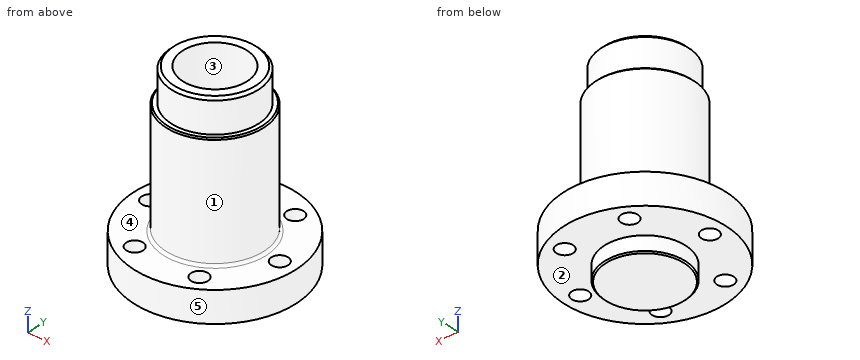
```python
from build123d import *

# Parameters (mm, degrees)
SKETCH1_R                  = 31.5
BOSS_EXTRUDE1_DEPTH        = 12
SKETCH3_R                  = 15.75
BOSS_EXTRUDE2_DEPTH        = 6
F_6_5_6_5_DIAMETER_HOLE1_D = 6.5
SKETCH14_R                 = 19
BOSS_EXTRUDE4_DEPTH        = 45
CHAMFER2_SIZE              = 0.5
FILLET3_R                  = 1
SKETCH15_R                 = 16.9375
BOSS_EXTRUDE6_DEPTH        = 13
CHAMFER3_SIZE              = 1
CHAMFER6_SIZE              = 0.5
F_25_0MM_DOWEL_HOLE1_D     = 25
F_25_0MM_DOWEL_HOLE1_DEPTH = 45
F_25_0MM_DOWEL_HOLE1_TIP   = 7.510757738


with BuildPart() as part:
    # Sketch1 → Boss-Extrude1 (new body)
    with BuildSketch(Plane.XY):
        Circle(SKETCH1_R)
    extrude(amount=BOSS_EXTRUDE1_DEPTH)

    # Sketch3 → Boss-Extrude2 (add)
    with BuildSketch(Plane(origin=(0, 0, 0), x_dir=(-1, 0, 0), z_dir=(0, 0, -1))):
        Circle(SKETCH3_R)
    extrude(amount=BOSS_EXTRUDE2_DEPTH)

    # Ø6.5 (6.5) Diameter Hole1 (through all)
    with Locations(Plane.XY.offset(12)):
        with Locations((-12.5, 21.650635095), (-25, 0), (-12.5, -21.650635095), (12.5, -21.650635095), (25, 0), (12.5, 21.650635095)):
            Hole(F_6_5_6_5_DIAMETER_HOLE1_D / 2)

    # Sketch14 → Boss-Extrude4 (add)
    with BuildSketch(Plane.XY.offset(12)):
        Circle(SKETCH14_R)
    extrude(amount=BOSS_EXTRUDE4_DEPTH)

    # Chamfer2
    chamfer2_edges = [part.edges().sort_by_distance(p)[0] for p in [
        (-19, 0, 57),
    ]]
    chamfer(chamfer2_edges, length=CHAMFER2_SIZE)

    # Fillet3
    fillet3_edges = [part.edges().sort_by_distance(p)[0] for p in [
        (-19, 0, 12),
    ]]
    fillet(fillet3_edges, radius=FILLET3_R)

    # Sketch15 → Boss-Extrude6 (add)
    with BuildSketch(Plane.XY.offset(57)):
        Circle(SKETCH15_R)
    extrude(amount=BOSS_EXTRUDE6_DEPTH)

    # Chamfer3
    chamfer3_edges = [part.edges().sort_by_distance(p)[0] for p in [
        (-16.9375, 0, 70),
    ]]
    chamfer(chamfer3_edges, length=CHAMFER3_SIZE)

    # Chamfer6
    chamfer6_edges = [part.edges().sort_by_distance(p)[0] for p in [
        (15.75, 0, -6),
    ]]
    chamfer(chamfer6_edges, length=CHAMFER6_SIZE)

    # Ø25.0mm Dowel Hole1
    with Locations(Plane.XY.offset(70)):
        with Locations((0, 0)):
            Hole(F_25_0MM_DOWEL_HOLE1_D / 2, depth=F_25_0MM_DOWEL_HOLE1_DEPTH)
            with Locations((0, 0, -(F_25_0MM_DOWEL_HOLE1_DEPTH + F_25_0MM_DOWEL_HOLE1_TIP / 2))):  # 118° drill point
                Cone(0, F_25_0MM_DOWEL_HOLE1_D / 2, F_25_0MM_DOWEL_HOLE1_TIP, mode=Mode.SUBTRACT)


solid = part.part
```
Geometry: final body of the model. Coordinates: model frame, mm. Face numbers are marked on the shaded views. A direction names the side the tool comes from. Give positions to 0.01 mm unless a question says otherwise; leave off trailing zeros. Order: outer loops, then holes, each group sorted by start corner. A loop starts at its lowest first (then second) coordinate and runs counter-clockwise, first axis right, second up. Notation, with made-up numbers: (33, 62) -> (79, 62) arc R15 ccw to (79, 77) -> close; hole circle Ø9 at (70, 4.25). An arc over 180 degrees is marked (long way). Write each question's results on one line, items separated by ' | '. Start each with the question number.
1) Draft query along X for the marked faces 1, 2 and 3. Return one class per face: pulls with the +X half, pulls with the -X half, needs draft (parallel to the pull), parting line crosses it, or undercut.
2) Set-up query: the marked faces 4 and 5. Return all of +Z, -Z, +X, -X, +Y, -Y with unobstructed straight access to the full face (end or side cutting, diameter ignored); none if empty.
3) First-contact query: pin 1 (6 mm diameter, centred on x = -18.5, y = -24, fed in from +Z); pin 2 (8 mm diameter, centred on y = 12, z = 37.5, fed in from +X); pin 3 (5 mm diameter, centred on x = -13.5, y = -21.5, fed in from -Z). Flat tips, straight axial feed; report the tip coordinate or a pass-through.
4) Section D-D (z = 16.5). Return loops of the section in (x, y).
5) Section C-C (z = 38.5). Return loops of the section in (x, y).
6) Section A-A (x = 25). Return loops of the section in (y, z), then the cut area to 3 significant figures.
7) Section B-B (z = 1). Return loops of the section in (x, y).
8) Line query: line 1 (Y direction, x = 13.5, z = 1); line 2 (Y direction, x = 0.5, z = 14.5); line 3 (Y direction, x = -12, z = 7). Output: solid intervals per line, ascending. Write a range as from..to.
Calculated:
1) face 1: parting line crosses it | face 2: needs draft | face 3: undercut
2) face 4: +Z | face 5: +Z, -Z
3) pin 1: z = 12 | pin 2: x = 17.23 | pin 3: z = 0
4) outline: circle Ø38 at (0, 0)
5) outline: circle Ø38 at (0, 0); hole circle Ø25 at (0, 0)
6) outline: (-19.16, 0) -> (-3.25, 0) -> (-3.25, 12) -> (-19.16, 12) -> close; (3.25, 0) -> (19.16, 0) -> (19.16, 12) -> (3.25, 12) -> close | area: 382 mm2
7) outline: circle Ø63 at (0, 0); hole circle Ø6.5 at (-25, 0); hole circle Ø6.5 at (-12.5, -21.65); hole circle Ø6.5 at (-12.5, 21.65); hole circle Ø6.5 at (12.5, -21.65); hole circle Ø6.5 at (12.5, 21.65); hole circle Ø6.5 at (25, 0)
8) line 1: -28.46..-24.74, -18.56..18.56, 24.74..28.46 | line 2: -18.99..18.99 | line 3: -29.12..-24.86, -18.44..18.44, 24.86..29.12
